Input: part model. Units: mm. Frame: model coordinates. A direction names the side the tool comes from. Give positions to 0.01 mm unless a question says otherwise; leave off trailing zeros. Loops run counter-clockwise (first coordinate to the right, second up) from the corner with the lowest first, then second, coordinate; pieces in that order, holes last. Notation, with made-up numbers: (-35, 47.5) - (14, 47.5) arc R15 cw to (14, 51.5) - close; hole circle Ø2 at (63.5, -24.5). An arc over 180 degrees is marked (long way). One line per item, written item: value.
from build123d import *

# Parameters (mm, degrees)
BOSS_EXTRUDE1_DEPTH = 19
SKETCH3_W           = 58
SKETCH3_H           = 58
BOSS_EXTRUDE2_DEPTH = 24
BOSS_EXTRUDE3_DEPTH = 66
SKETCH6_W           = 28
SKETCH6_H           = 14
BOSS_EXTRUDE4_DEPTH = 25.1
SKETCH7_W           = 64
SKETCH7_H           = 304.8
BOSS_EXTRUDE5_DEPTH = 6.35
SKETCH8_R           = 3
CUT_EXTRUDE1_DEPTH  = 5


with BuildPart() as part:
    # Sketch2 → Boss-Extrude1 (new body)
    with BuildSketch(Plane(origin=(0, 0, 0), x_dir=(1, 0, 0), z_dir=(0, 1, 0))):
        with BuildLine():
            Line((5, 0), (59, 0))
            ThreePointArc((59, 0), (62.535533906, -1.464466094), (64, -5))
            Line((64, -5), (64, -59))
            ThreePointArc((64, -59), (62.535533906, -62.535533906), (59, -64))
            Line((59, -64), (5, -64))
            ThreePointArc((5, -64), (1.464466094, -62.535533906), (0, -59))
            Line((0, -59), (0, -5))
            ThreePointArc((0, -5), (1.464466094, -1.464466094), (5, 0))
        make_face()
    extrude(amount=BOSS_EXTRUDE1_DEPTH)

    # Sketch3 → Boss-Extrude2 (add)
    with BuildSketch(Plane(origin=(0, 19, 0), x_dir=(1, 0, 0), z_dir=(0, 1, 0))):
        with Locations((32, -32)):
            Rectangle(SKETCH3_W, SKETCH3_H)
    extrude(amount=BOSS_EXTRUDE2_DEPTH)

    # Sketch4 → Boss-Extrude3 (add)
    with BuildSketch(Plane(origin=(0, 43, 0), x_dir=(1, 0, 0), z_dir=(0, 1, 0))):
        with BuildLine():
            Line((5, 0), (59, 0))
            ThreePointArc((59, 0), (62.535533906, -1.464466094), (64, -5))
            Line((64, -5), (64, -58.999541839))
            ThreePointArc((64, -58.999541839), (62.535533906, -62.535075745), (59, -63.999541839))
            Line((59, -63.999541839), (5, -63.999541839))
            ThreePointArc((5, -63.999541839), (1.464466094, -62.535075745), (0, -58.999541839))
            Line((0, -58.999541839), (0, -5))
            ThreePointArc((0, -5), (1.464466094, -1.464466094), (5, 0))
        make_face()
    extrude(amount=BOSS_EXTRUDE3_DEPTH)

    # Sketch6 → Boss-Extrude4 (add)
    with BuildSketch(Plane.ZY):
        with Locations((32, 9)):
            Rectangle(SKETCH6_W, SKETCH6_H)
    extrude(amount=BOSS_EXTRUDE4_DEPTH)

    # Sketch7 → Boss-Extrude5 (add)
    with BuildSketch(Plane(origin=(0, 109, 0), x_dir=(1, 0, 0), z_dir=(0, 1, 0))):
        with Locations((32, -32)):
            Rectangle(SKETCH7_W, SKETCH7_H)
    extrude(amount=BOSS_EXTRUDE5_DEPTH)

    # Sketch8 → Cut-Extrude1 (cut)
    with BuildSketch(Plane(origin=(0, 115.35, 0), x_dir=(1, 0, 0), z_dir=(0, 1, 0))):
        with BuildLine():
            ThreePointArc((7, -10), (9.121320344, -9.121320344), (10, -7))
            Line((10, -7), (7, -7))
            Line((7, -7), (7, -10))
        make_face()
        with BuildLine():
            Line((7, -7), (10, -7))
            ThreePointArc((10, -7), (4.878679656, -4.878679656), (7, -10))
            Line((7, -10), (7, -7))
        make_face()
        with Locations((57, -7)):
            Circle(SKETCH8_R)
        with Locations((57, -57)):
            Circle(SKETCH8_R)
        with Locations((7, -57)):
            Circle(SKETCH8_R)
    extrude(amount=-CUT_EXTRUDE1_DEPTH, mode=Mode.SUBTRACT)


solid = part.part
Item 1: Section C-C, the plane x = 21. Output: boundary loops of the cut face in (y, z), and give its area (3 significant figures).
Verdict:
outline: (0, 0) - (19, 0) - (19, 3) - (43, 3) - (43, 0) - (109, 0) - (109, -120.4) - (115.35, -120.4) - (115.35, 184.4) - (109, 184.4) - (109, 64) - (43, 64) - (43, 61) - (19, 61) - (19, 64) - (0, 64) - close
area: 8,770 mm^2
Item 2: Section B-B, the plane z = 51. Output: boundary loops of the cut face in (x, y).
Verdict:
outline: (0, 0) - (64, 0) - (64, 19) - (61, 19) - (61, 43) - (64, 43) - (64, 115.35) - (0, 115.35) - (0, 43) - (3, 43) - (3, 19) - (0, 19) - close
Item 3: Pin query (flat end, axial travel): P1, Ø10, axis at x = 47, y = 39, coming from the +Z side; P2, Ø6, axis at x = 0, y = 73, coming from the -Z side; P3, Ø12, axis at x = -8, y = 97, coming from the +Z side; P4, Ø3, axis at x = 8, z = 56, coming from the +Y side. Return the tip coordinate at first contact, or that it passes through.
Verdict:
P1: stops at z = 64
P2: stops at z = 0.42
P3: passes through
P4: stops at y = 110.35
Item 4: Section A-A, the plane y = 93.5. Output: boundary loops of the cut face in (x, z).
Verdict:
outline: (0, 5) arc R5 ccw to (5, 0) - (59, 0) arc R5 ccw to (64, 5) - (64, 59) arc R5 ccw to (59, 64) - (5, 64) arc R5 ccw to (0, 59) - close
Item 5: Section D-D, the plane y = 13. Output: boundary loops of the cut face in (x, z).
Verdict:
outline: (-25.1, 18) - (0, 18) - (0, 5) arc R5 ccw to (5, 0) - (59, 0) arc R5 ccw to (64, 5) - (64, 59) arc R5 ccw to (59, 64) - (5, 64) arc R5 ccw to (0, 59) - (0, 46) - (-25.1, 46) - close
Item 6: Material intervals for L1, parallel to X at y = 111, z = 57; L2, parallel to Z at x = 7, y = 111; L3, parallel to Y at x = 22.5, z = -27.5, sorted ascending.
Verdict:
L1: x = 0 to 4, 10 to 54, 60 to 64
L2: z = -120.4 to 4, 10 to 54, 60 to 184.4
L3: y = 109 to 115.35
Item 7: Draft query along X for faces 1 (the face through (64, 9, 32)), 2 (the face through (32, 109, 121)), 3 (the face through (57, 110.35, 7)). Return one class per face: pulls with the +X half, pulls with the -X half, needs draft (parallel to the pull), parting line crosses it, or undercut.
Verdict:
face 1: pulls with the +X half
face 2: needs draft
face 3: undercut
Item 8: Access query for faces 4 (the face through (54.79, 112.88, 54.97)), 5 (the face through (-12, 9, 18)), 6 (the face through (0, 87, 33)). Directions: +Z, -Z, +X, -X, +Y, -Y. A direction counts if a zero-diameter tool reaches every point of the face in a straight line with its end or side. Return the directions, or none.
Verdict:
face 4: +Y
face 5: -Z, -X, +Y, -Y
face 6: +Z, -Z, -X, +Y
